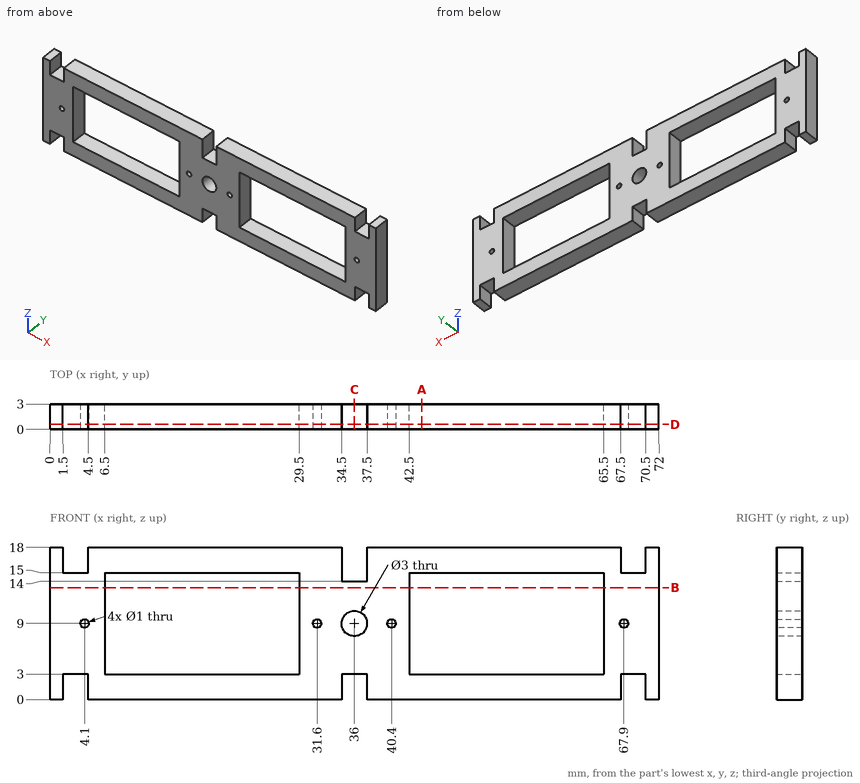
Print and shaded views of the part. All mm, measured from the part's lowest x, y and z. Coordinates: 2 decimals unless noted, no trailing zeros. Write each loop counter-clockwise with the first axis right and the second up, starting at its lowest first coordinate (ties: lowest second). Pieces come first, ordered by that corner, then holes. Notation, with made-up numbers: (65.25, -20.5) - (108.25, -20.5) arc R30 cw to (108.25, 5.5) - close; hole circle Ø11 at (-5, -7.75). An arc over 180 degrees is marked (long way). One line per question, with ' | ' between items. Start each with the question number.
Q1. Drill centre lines: line 1 (X direction, y = 0.55, z = 11.75); line 2 (X direction, y = 1.2, z = 14.5); line 3 (X direction, y = 0.7, z = 2). Where is each one in solid material? Low to high. Write a range as [from, to].
Q2. Cut at C-C, the plane x = 36. List the corners of the cut face in (y, z).
Q3. Cut at B-B, the plane z = 13.25. List the corners of the cut face in (x, y).
Q4. Cut at A-A, the plane x = 44. List the corners of the cut face in (y, z).
Q5. Pin check, flat tips, straight feed: pin 1 (0.9 mm diameter, centred on x = 2.5, y = 1.5, fed in from +Z); pin 2 (2 mm diameter, centred on x = 21, z = 14.5, fed in from +Y); pin 3 (1.5 mm diameter, centred on x = 36.5, y = 1.5, fed in from +Z). Stop position of each tip, or through.
Q6. Cut at D-D, the plane y = 0.6. Give the number of separate pieces and of enclosed holes in the cut face, then the cut area to 3 significant figures.
Answer below:
1) line 1: [0, 6.5], [29.5, 42.5], [65.5, 72] | line 2: [0, 6.5], [29.5, 34.5], [37.5, 42.5], [65.5, 72] | line 3: [0, 1.5], [4.5, 34.5], [37.5, 67.5], [70.5, 72]
2) outline: (0, 3) - (3, 3) - (3, 7.5) - (0, 7.5) - close; (0, 10.5) - (3, 10.5) - (3, 14) - (0, 14) - close
3) outline: (0, 0) - (6.5, 0) - (6.5, 3) - (0, 3) - close; (29.5, 0) - (42.5, 0) - (42.5, 3) - (29.5, 3) - close; (65.5, 0) - (72, 0) - (72, 3) - (65.5, 3) - close
4) outline: (0, 0) - (3, 0) - (3, 3) - (0, 3) - close; (0, 15) - (3, 15) - (3, 18) - (0, 18) - close
5) pin 1: z = 15 | pin 2: y = 3 | pin 3: z = 14
6) separate pieces: 1 | enclosed holes: 7 | area: 677 mm^2
